from build123d import *

# Parameters (mm, degrees)
SCHIZZO1_R                   = 1.5
ESTRUSIONE_ESTRUSIONE1_DEPTH = 4
SCHIZZO2_R                   = 1.5
TAGLIO_ESTRUSIONE1_DEPTH     = 25


with BuildPart() as part:
    # Schizzo1 → Estrusione-Estrusione1 (new body)
    with BuildSketch(Plane.XY):
        with BuildLine():
            ThreePointArc((7.023974797, 138.427683332), (1.499753731, 147.278176914), (-7.525391936, 142.044153534))
            ThreePointArc((-7.525391936, 142.044153534), (-18.729107246, 69.99949188), (-12.22229981, -2.620188418))
            ThreePointArc((-12.22229981, -2.620188418), (3.068449146, -12.117533571), (11.996332959, 3.512548298))
            ThreePointArc((11.996332959, 3.512548298), (1.102237583, 70.660238267), (7.023974797, 138.427683332))
        make_face()
        Circle(SCHIZZO1_R, mode=Mode.SUBTRACT)
        with Locations((-0.309434746, 139.999658036)):
            Circle(SCHIZZO1_R, mode=Mode.SUBTRACT)
    extrude(amount=ESTRUSIONE_ESTRUSIONE1_DEPTH)

    # Schizzo2 → Taglio-Estrusione1 (cut)
    with BuildSketch(Plane.XY.offset(4)):
        with Locations((-6.142115432, 104.166670735)):
            Circle(SCHIZZO2_R)
        with Locations((-6.142115432, 32.213749463)):
            Circle(SCHIZZO2_R)
    extrude(amount=-TAGLIO_ESTRUSIONE1_DEPTH, mode=Mode.SUBTRACT)


solid = part.part
The listing builds one solid part. Answer for the finished solid, in the listing's coordinates (mm). Give positions to 0.01 mm unless a question says otherwise; leave off trailing zeros. Loops run counter-clockwise (first coordinate to the right, second up) from the corner with the lowest first, then second, coordinate; pieces in that order, holes last.
Item 1: A cutting plane is placed at A-A (y = 0). Give the vertices of the cut face in (x, z), then the cut area to 3 significant figures.
Derived:
outline: (-12.77, 0) - (-1.5, 0) - (-1.5, 4) - (-12.77, 4) - close; (1.5, 0) - (12.5, 0) - (12.5, 4) - (1.5, 4) - close
area: 89.1 mm2
Item 2: Determine the mould class of faces 1 (the flat face through (-7, 69, 0)), 2 (the cylindrical face through (-18.694, 71.022, 1.972)), 3 (the cylindrical face through (-5.45, 30.883, 2.028)) for opening direction X: +X half, -X half, draft (parallel to the pull), parting line (faces both ways), or undercut.
Derived:
face 1: draft
face 2: -X half
face 3: undercut
Item 3: A cutting plane is placed at C-C (z = 1.05). Give the vertices of the cut face in (x, y).
Derived:
outline: (-12.22, -2.62) arc R12.5 ccw (long way) to (12, 3.51) arc R275 cw to (7.02, 138.43) arc R7.5 ccw to (-7.53, 142.04) arc R300 ccw to start; hole circle Ø3 at (-6.14, 32.21); hole circle Ø3 at (-6.14, 104.17); hole circle Ø3 at (-0.31, 140); hole circle Ø3 at (0, 0)
Item 4: A cutting plane is placed at D-D (y = 79.5). Give the vertices of the cut face in (x, z), then the cut area to 3 significant figures.
Derived:
outline: (-18.27, 0) - (0.92, 0) - (0.92, 4) - (-18.27, 4) - close
area: 76.8 mm2
Item 5: A cutting plane is placed at B-B (x = 4). Give the vertices of the cut face in (y, z), then the cut area to 3 significant figures.
Derived:
outline: (-11.84, 0) - (39.72, 0) - (39.72, 4) - (-11.84, 4) - close; (121.86, 0) - (146.14, 0) - (146.14, 4) - (121.86, 4) - close
area: 303 mm2
Item 6: Each of these flat-tipped pins is pushed along its axis until it touches: pin 1 Ø3.5 at (x, y) = (-6.14, 104.17) entering from -Z; pin 2 Ø1.5 at (x, y) = (2.5, 66.5) entering from -Z; pin 3 Ø2 at (y, z) = (5, 3) entering from +X. Where does it stop, or does it pass through?
Derived:
pin 1: stops at z = 0
pin 2: passes through
pin 3: stops at x = 11.85
Item 7: Find the intervals of material crossed by line 1 along Y through (x, z) = (0, 1); line 2 along X through (y, z) = (133.5, 3.55); line 3 along X through (y, z) = (60, 1.7), in increasing order.
Derived:
line 1: y = -12.5 to -1.5, 1.5 to 138.53, 141.47 to 147.49
line 2: x = -9.81 to 6.01
line 3: x = -18.89 to 1.7
